Work out the finished part from the listing and answer in its coordinate system (mm). Round coordinates to 2 decimals unless told otherwise and drop trailing zeros. Loops run counter-clockwise (first coordinate to the right, second up) from the corner with the lowest first, then second, coordinate; pieces in that order, holes last. Notation, with made-up numbers: M 44,9 L 88,9 A24 cw 88,24 Z; hole C 15.25,0 d3. An arc over 180 degrees is marked long. One line per item, written item: value.
```python
from build123d import *

# Parameters (mm, degrees)
SKETCH1_W           = 28
SKETCH1_H           = 28
BOSS_EXTRUDE1_DEPTH = 15
SKETCH2_W           = 15
SKETCH2_H           = 7
BOSS_EXTRUDE2_DEPTH = 1.5
FILLET1_R           = 3


with BuildPart() as part:
    # Sketch1 → Boss-Extrude1 (new body, symmetric)
    with BuildSketch(Plane.XY):
        Rectangle(SKETCH1_W, SKETCH1_H)
    extrude(amount=BOSS_EXTRUDE1_DEPTH, both=True)

    # Sketch2 → Boss-Extrude2 (add, symmetric)
    with BuildSketch(Plane.XZ.offset(14)):
        with Locations((0, -11.5)):
            Rectangle(SKETCH2_W, SKETCH2_H)
    extrude(amount=BOSS_EXTRUDE2_DEPTH, both=True)

    # Fillet1
    fillet1_edges = [part.edges().sort_by_distance(p)[0] for p in [
        (14, -14, 0),
        (-14, -14, 0),
        (-14, 14, 0),
        (14, 14, 0),
    ]]
    fillet(fillet1_edges, radius=FILLET1_R)


solid = part.part
```
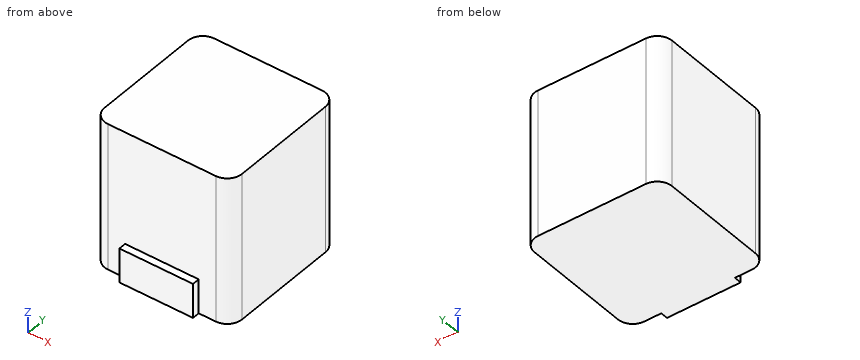
1) Each of these flat-tipped pins is pushed along its axis until it touches: pin 1 (3 mm diameter, centred on x = 2.5, z = 5, fed in from -Y); pin 2 (0.8 mm diameter, centred on x = 1.5, y = -15, fed in from +Z). Where does it stop, or does it pass through?
Check values:
pin 1: y = -14
pin 2: z = -8
2) Find section B-B (x = -2). Give the vertices of the cut face in (y, z), then the cut area to 4 significant figures.
Check values:
outline: M -15.5,-15 L 14,-15 L 14,15 L -14,15 L -14,-8 L -15.5,-8 Z
area: 850.5 mm2
3) Find section A-A (z = -11). Give the vertices of the cut face in (x, y).
Check values:
outline: M -14,-11 A3 ccw -11,-14 L -7.5,-14 L -7.5,-15.5 L 7.5,-15.5 L 7.5,-14 L 11,-14 A3 ccw 14,-11 L 14,11 A3 ccw 11,14 L -11,14 A3 ccw -14,11 Z
4) Find section C-C (z = 7.75). Give the vertices of the cut face in (x, y), then the cut area to 3 significant figures.
Check values:
outline: M -14,-11 A3 ccw -11,-14 L 11,-14 A3 ccw 14,-11 L 14,11 A3 ccw 11,14 L -11,14 A3 ccw -14,11 Z
area: 776 mm2
5) Find the intervals of material crossed by probe 1 along Y at (x, z) = (-11, -7.75); probe 2 along X at (y, z) = (-13.75, 11.5); probe 3 along Y at (x, z) = (12, -3.25), in increasing order. Write a range as from..to.
Check values:
probe 1: -14..14
probe 2: -12.2..12.2
probe 3: -13.83..13.83
